Autodesk Inventor part; units mm, degrees
ref_plane "YZ Plane" through (0, 0, 0) normal (1, 0, 0) x (0, 1, 0)
ref_plane "XZ Plane" through (0, 0, 0) normal (0, 1, 0) x (-1, 0, 0)
ref_plane "XY Plane" through (0, 0, 0) normal (0, 0, 1) x (1, 0, 0)
sketch "スケッチ1" plane through (0, 0, 0) normal (0, 0, 1) x (1, 0, 0)
  line L0 (-25, 9.4) -> (25, 9.4)
  line L1 (25, 9.4) -> (25, -9.4)
  line L2 (25, -9.4) -> (-25, -9.4)
  line L3 (-25, -9.4) -> (-25, 9.4)
  line L4 (25, 0) -> (-25, 0)
  circle A0 centre (11.2, 4.4) radius 1
  circle A1 centre (20, 4.4) radius 1
  circle A2 centre (11.2, -4.4) radius 1
  circle A3 centre (20, -4.4) radius 1
  point P0 (0, 0)
  dimension "d0" = 50
  dimension "d1" = 18.8
  dimension "d2" = 9.4
  dimension "d3" = 25
  dimension "d4" = 8.8
  dimension "d5" = 8.8
  dimension "d6" = 8.8
  dimension "d7" = 8.8
  dimension "d8" = 8.8
  dimension "d9" = 5
  dimension "d10" = 2
  dimension "d11" = 2
  dimension "d12" = 2
  dimension "d13" = 2
extrude "押し出し1" add sketch "スケッチ1" along normal blind 5
fillet "フィレット1" radius 9.4 2 edges at (25, 9.4, 2.5) (25, -9.4, 2.5)
sketch "スケッチ2" plane through (0, 0, 5) normal (0, 0, 1) x (1, 0, 0)
  arc A0 (15.6, -9.4) -> (15.6, 9.4) centre (15.6, 0) ccw
  circle A1 centre (15.6, 0) radius 4.25
  point P0 (0, 0)
  dimension "d17" = 8.5
extrude "押し出し2" cut sketch "スケッチ2" against normal through all
mirror "ミラー1" about plane through (-25, 0, 0) normal (-1, 0, 0)
sketch "スケッチ3" plane through (0, 0, 5) normal (0, 0, 1) x (1, 0, 0)
  arc A0 (15.6, -9.4) -> (15.6, 9.4) centre (15.6, 0) ccw
  line L0 (-65.6, 9.4) -> (15.6, 9.4)
  arc A1 (-65.6, 9.4) -> (-65.6, -9.4) centre (-65.6, 0) ccw
  line L1 (-65.6, 0) -> (15.6, 0)
  circle A2 centre (11.2, -4.4) radius 1
  point P0 (0, 0)
  point P1 (-18.8, 4.4)
  point P2 (-18.8, -4.4)
  point P3 (-8.8, 0)
  dimension "d20" = 8.8
  dimension "d32" = 20
  dimension "d33" = 4.4
  dimension "d34" = 10
  dimension "d35" = 10
hole "Hole1" at (-18.8, 4.4, 5) at (-18.8, -4.4, 5) at (-8.8, 0, 5) direction (0, 0, -1) diameter 3.2 depth 8 tip angle 118
properties part number "JointC4"
Read the model definition and answer for the solid it produces. Units are mm, in the model's axes. Round coordinates to 2 decimals unless told otherwise and drop trailing zeros. Write each loop counter-clockwise with the first axis right and the second up, starting at its lowest first coordinate (ties: lowest second). Pieces come first, ordered by that corner, then holes. Notation, with made-up numbers: (57.5, 70) - (107.5, 70) arc R19 cw to (107.5, 77) - close; hole circle Ø8 at (32, -29). An arc over 180 degrees is marked (long way). One line per item, written item: value.
Q1. Find section A-A (x = -18.8). Determine the outline of the cut face in (y, z), and give its area (3 significant figures).
The answers:
outline: (-9.4, 0) - (-6, 0) - (-6, 5) - (-9.4, 5) - close; (-2.8, 0) - (2.8, 0) - (2.8, 5) - (-2.8, 5) - close; (6, 0) - (9.4, 0) - (9.4, 5) - (6, 5) - close
area: 62.0 mm2
Q2. For a pull along X with two mould halves and no side action, classify faces 1 (the flat face through (-26, 0, 5)), 2 (the cylindrical face through (-17.24, 4.75, 2.46)), 3 (the cylindrical face through (-69, -4.4, 2.5)), 4 (the cylindrical face through (-72.32, -6.57, 2.54)) as pulls with the +X half, pulls with the -X half, needs draft (parallel to the pull), parting line crosses it, or undercut.
The answers:
face 1: needs draft
face 2: undercut
face 3: undercut
face 4: pulls with the -X half
Q3. Find section C-C (y = -8). Determine the outline of the cut face in (x, z).
The answers:
outline: (-70.54, 0) - (20.54, 0) - (20.54, 5) - (-70.54, 5) - close
Q4. Each of these flat-tipped pins is pushed along its axis until it touches: P1, Ø3, axis at y = -3, z = 1.5, coming from the -X side; P2, Ø1.5, axis at y = 5.5, z = 2, coming from the -X side. Where does it stop, or does it pass through?
The answers:
P1: stops at x = -74.88
P2: stops at x = -73.71
Q5. Find section B-B (z = 2.9). Count the separate pieces of the cut face and the enclosed holes in it, and give its area (3 significant figures).
The answers:
separate pieces: 1
enclosed holes: 13
area: 1,640 mm2
Q6. Straight lines are drawn through the part: line 1 (Y direction, x = -19, z = 1.7); line 2 (Y direction, x = -61.2, z = 2.8); line 3 (X direction, y = 3, z = 2.6). For each, find the intervals that lie inside material, in ascending order. Write a range as from..to.
The answers:
line 1: y = -9.4..-5.99, -2.81..2.81, 5.99..9.4
line 2: y = -9.4..-5.4, -3.4..3.4, 5.4..9.4
line 3: x = -74.51..-68.61, -62.59..-19.57, -18.03..12.59, 18.61..24.51
